Autodesk Inventor part; units mm, degrees
ref_plane "YZ Plane" through (0, 0, 0) normal (1, 0, 0) x (0, 1, 0)
ref_plane "XZ Plane" through (0, 0, 0) normal (0, 1, 0) x (-1, 0, 0)
ref_plane "XY Plane" through (0, 0, 0) normal (0, 0, 1) x (1, 0, 0)
sketch "Skizze6" plane through (0, 0, 0) normal (0, 0, 1) x (1, 0, 0)
  arc A0 (21.4454, -27.1023) -> (20.0312, -26.5165) centre (20.0312, -28.5165) ccw
  line L0 (20.0312, -26.5165) -> (-20.0312, -26.5165)
  arc A1 (-20.0312, -26.5165) -> (-21.4454, -27.1023) centre (-20.0312, -28.5165) ccw
  line L1 (-21.4454, -27.1023) -> (-51.9723, -57.6292)
  line L2 (-51.9723, -57.6292) -> (-42.4264, -67.1751)
  arc A2 (-38.3776, -89.6293) -> (-42.4264, -67.1751) centre (-56.5685, -81.3173) ccw
  arc A3 (-38.3776, -89.6293) -> (38.3776, -89.6293) centre (0, 0) ccw
  arc A4 (42.4264, -67.1751) -> (38.3776, -89.6293) centre (56.5685, -81.3173) ccw
  line L3 (42.4264, -67.1751) -> (51.9724, -57.6292)
  line L4 (51.9724, -57.6292) -> (21.4454, -27.1023)
  circle A5 centre (37.8302, -37.8302) radius 1.65
  circle A6 centre (37.8302, 37.8302) radius 1.65
  circle A7 centre (-37.8302, -37.8302) radius 1.65
  circle A8 centre (-37.8302, 37.8302) radius 1.65
  circle A9 centre (-22.7665, 22.7665) radius 1.6
  circle A10 centre (22.7665, 22.7665) radius 1.6
  circle A11 centre (22.7665, -22.7665) radius 1.6
  circle A12 centre (-22.7665, -22.7665) radius 1.6
  line L5 (19.0165, -19.0165) -> (19.0165, 19.0165)
  line L6 (19.0165, 19.0165) -> (-19.0165, 19.0165)
  line L7 (-19.0165, 19.0165) -> (-19.0165, -19.0165)
  line L8 (-19.0165, -19.0165) -> (19.0165, -19.0165)
  line L9 (26.5165, -20.8596) -> (57.6292, -51.9723)
  line L10 (57.6292, -51.9723) -> (67.1751, -42.4264)
  arc A13 (89.6293, -38.3776) -> (67.1751, -42.4264) centre (81.3173, -56.5685) ccw
  arc A14 (89.6293, -38.3776) -> (89.6293, 38.3776) centre (0, 0) ccw
  arc A15 (67.1751, 42.4264) -> (89.6293, 38.3776) centre (81.3173, 56.5685) ccw
  line L11 (67.1751, 42.4264) -> (57.6292, 51.9724)
  line L12 (57.6292, 51.9724) -> (26.5165, 20.8597)
  line L13 (26.5165, 20.8597) -> (26.5165, -20.8596)
  line L14 (-26.5165, 20.8596) -> (-57.6292, 51.9723)
  line L15 (-57.6292, 51.9723) -> (-67.1751, 42.4264)
  arc A16 (-89.6293, 38.3776) -> (-67.1751, 42.4264) centre (-81.3173, 56.5685) ccw
  arc A17 (-89.6293, 38.3776) -> (-89.6293, -38.3776) centre (0, 0) ccw
  arc A18 (-67.1751, -42.4264) -> (-89.6293, -38.3776) centre (-81.3173, -56.5685) ccw
  line L16 (-67.1751, -42.4264) -> (-57.6292, -51.9724)
  line L17 (-57.6292, -51.9724) -> (-26.5165, -20.8597)
  line L18 (-26.5165, -20.8597) -> (-26.5165, 20.8596)
  circle A19 centre (-44.3776, -92.6293) radius 1.6
  circle A20 centre (92.6293, 44.3776) radius 1.6
  circle A21 centre (-92.6293, -44.3776) radius 1.6
  circle A22 centre (44.3776, -92.6293) radius 1.6
  circle A23 centre (92.6293, -44.3776) radius 1.6
  circle A24 centre (-92.6293, 44.3776) radius 1.6
  circle A25 centre (45, 91.781) radius 1.6
  circle A26 centre (-45, 91.781) radius 1.6
  circle A27 centre (-67.8822, -48.7904) radius 1.6
  circle A28 centre (-48.7904, -67.8823) radius 1.6
  circle A29 centre (48.7904, -67.8822) radius 1.6
  circle A30 centre (67.8823, -48.7904) radius 1.6
  circle A31 centre (-67.8823, 48.7904) radius 1.6
  circle A32 centre (67.8822, 48.7904) radius 1.6
  circle A33 centre (48.7904, 67.8823) radius 1.6
  circle A34 centre (-48.7904, 67.8822) radius 1.6
  arc A35 (12, 61.781) -> (38.5642, 72.6085) centre (12, 99.781) ccw
  line L19 (12, 61.781) -> (-12, 61.781)
  arc A36 (-38.5642, 72.6085) -> (-12, 61.781) centre (-12, 99.781) ccw
  arc A37 (-42.4264, 67.1751) -> (-38.5642, 72.6085) centre (-56.5685, 81.3173) ccw
  line L20 (-42.4264, 67.1751) -> (-51.9724, 57.6292)
  line L21 (-51.9724, 57.6292) -> (-20.8597, 26.5165)
  line L22 (-20.8597, 26.5165) -> (20.8596, 26.5165)
  line L23 (20.8596, 26.5165) -> (51.9723, 57.6292)
  line L24 (51.9723, 57.6292) -> (42.4264, 67.1751)
  arc A38 (38.5642, 72.6085) -> (42.4264, 67.1751) centre (56.5685, 81.3173) ccw
  line L25 (-12, 71.781) -> (12, 71.781)
  arc A39 (12, 71.781) -> (39.8653, 97.0378) centre (12, 99.781) ccw
  arc A40 (42.6492, 98.6778) -> (39.8653, 97.0378) centre (41.8557, 96.8419) ccw
  arc A41 (50.5184, 94.8902) -> (42.6492, 98.6778) centre (0, 0) ccw
  arc A42 (51.2299, 90.1207) -> (50.5184, 94.8902) centre (49.1086, 92.2421) ccw
  line L26 (51.2299, 90.1207) -> (49.4975, 88.3883)
  arc A43 (49.4975, 88.3883) -> (49.4975, 74.2462) centre (56.5685, 81.3173) ccw
  line L27 (49.4975, 74.2462) -> (74.2462, 49.4975)
  arc A44 (74.2462, 49.4975) -> (88.3884, 49.4975) centre (81.3173, 56.5685) ccw
  line L28 (88.3884, 49.4975) -> (90.1208, 51.2299)
  arc A45 (94.8902, 50.5184) -> (90.1208, 51.2299) centre (92.2421, 49.1086) ccw
  arc A46 (94.8902, -50.5184) -> (94.8902, 50.5184) centre (0, 0) ccw
  arc A47 (90.1208, -51.2299) -> (94.8902, -50.5184) centre (92.2421, -49.1086) ccw
  line L29 (90.1208, -51.2299) -> (88.3883, -49.4975)
  arc A48 (88.3883, -49.4975) -> (74.2462, -49.4975) centre (81.3173, -56.5685) ccw
  line L30 (74.2462, -49.4975) -> (49.4975, -74.2462)
  arc A49 (49.4975, -74.2462) -> (49.4975, -88.3883) centre (56.5685, -81.3173) ccw
  line L31 (49.4975, -88.3883) -> (51.2299, -90.1207)
  arc A50 (50.5184, -94.8902) -> (51.2299, -90.1207) centre (49.1086, -92.2421) ccw
  arc A51 (-50.5184, -94.8902) -> (50.5184, -94.8902) centre (0, 0) ccw
  arc A52 (-51.2299, -90.1208) -> (-50.5184, -94.8902) centre (-49.1086, -92.2421) ccw
  line L32 (-51.2299, -90.1208) -> (-49.4975, -88.3883)
  arc A53 (-49.4975, -88.3883) -> (-49.4975, -74.2462) centre (-56.5685, -81.3173) ccw
  line L33 (-49.4975, -74.2462) -> (-74.2462, -49.4975)
  arc A54 (-74.2462, -49.4975) -> (-88.3883, -49.4975) centre (-81.3173, -56.5685) ccw
  line L34 (-88.3883, -49.4975) -> (-90.1207, -51.2299)
  arc A55 (-94.8902, -50.5184) -> (-90.1207, -51.2299) centre (-92.2421, -49.1086) ccw
  arc A56 (-94.8902, 50.5184) -> (-94.8902, -50.5184) centre (0, 0) ccw
  arc A57 (-90.1208, 51.2299) -> (-94.8902, 50.5184) centre (-92.2421, 49.1086) ccw
  line L35 (-90.1208, 51.2299) -> (-88.3883, 49.4975)
  arc A58 (-88.3883, 49.4975) -> (-74.2462, 49.4975) centre (-81.3173, 56.5685) ccw
  line L36 (-74.2462, 49.4975) -> (-49.4975, 74.2462)
  arc A59 (-49.4975, 74.2462) -> (-49.4975, 88.3883) centre (-56.5685, 81.3173) ccw
  line L37 (-49.4975, 88.3883) -> (-51.2299, 90.1207)
  arc A60 (-50.5184, 94.8902) -> (-51.2299, 90.1207) centre (-49.1086, 92.2421) ccw
  arc A61 (-42.6492, 98.6778) -> (-50.5184, 94.8902) centre (0, 0) ccw
  arc A62 (-39.8653, 97.0378) -> (-42.6492, 98.6778) centre (-41.8557, 96.8419) ccw
  arc A63 (-39.8653, 97.0378) -> (-12, 71.781) centre (-12, 99.781) ccw
  arc A64 (-47.6003, 86.4911) -> (-12, 61.781) centre (-12, 99.781) ccw
  line L38 (-49.4975, 88.3883) -> (-47.6003, 86.4911)
  line L39 (0, 71.781) -> (0, 61.781) construction
  arc A65 (12, 61.781) -> (47.6003, 86.4911) centre (12, 99.781) ccw
  line L40 (49.4975, 88.3883) -> (47.6003, 86.4911)
  point P0 (0, 0)
  point P1 (0, 0)
  point P2 (38.5642, 72.6085)
extrude "Extrusion4" add sketch "Skizze6" against normal blind 30 contours L19 A36 A64 L38 L37 A60 A61 A62 A63 L25 A39 A40 A41 A42 L26 L40 A65 A35
fillet "Rundung2" radius 20 2 edges at (47.6003, 86.4911, -15) (-47.6003, 86.4911, -15)
sketch "Skizze7" plane through (0, 0, 0) normal (0, 0, 1) x (1, 0, 0)
  line L0 (0, 0) -> (-29.0841, 0) construction
  line L1 (0, 0) -> (-84.8528, 84.8528)
  line L2 (-111.3693, 68.9429) -> (-68.9429, 111.3693)
  line L3 (-68.9429, 111.3693) -> (-58.3363, 100.7627)
  line L4 (-58.3363, 100.7627) -> (-100.7627, 58.3363)
  line L5 (-100.7627, 58.3363) -> (-111.3693, 68.9429)
  line L6 (-111.3693, 68.9429) -> (-58.3363, 100.7627) construction
  line L7 (-68.9429, 111.3693) -> (-100.7627, 58.3363) construction
  dimension "d19" = 45
  dimension "d20" = 120
  dimension "d21" = 60
  dimension "d22" = 15
extrude "Extrusion5" add sketch "Skizze7" against normal blind 30
sketch "Skizze8" plane through (-68.9429, 111.3693, -30) normal (-0.7071, 0.7071, 0) x (-0.7071, -0.7071, 0)
  line L0 (60, 0) -> (0, 0)
  line L1 (30, 0) -> (30, 17.5)
  circle A0 centre (30, 17.5) radius 30
  line L2 (0, 30) -> (60, 30)
  line L3 (0, 30) -> (60, 30)
  line L4 (60, 30) -> (60, 0)
  line L5 (60, 0) -> (0, 0)
  line L6 (0, 0) -> (0, 30)
  point P0 (30, 30)
  dimension "d25" = 17.5
  dimension "d26" = 60
extrude "Extrusion6" cut sketch "Skizze8" against normal up to surface (15 mm away) contours L0 A0 L4 | L0 A0 L2 | A0 L2 L4 | L0 L6 A0 | L6 L2 A0
extrude "Extrusion7" cut sketch "Skizze8" against normal blind 100 contours A0 L0 | L0 A0 L2 | L2 A0
mirror "Spiegeln1" about plane through (0, 0, 0) normal (1, 0, 0) of "Extrusion7"
sketch "Skizze9" plane through (0, 0, 0) normal (0, 0, 1) x (1, 0, 0)
  circle A0 centre (45, 91.781) radius 1.6
  circle A1 centre (45, 91.781) radius 2.1
  circle A2 centre (-45, 91.781) radius 1.6
  circle A3 centre (-45, 91.781) radius 2.1
  point P0 (0, 0)
  dimension "d31" = 4.2
  dimension "d32" = 4.2
extrude "Extrusion8" cut sketch "Skizze9" against normal up to surface (30 mm away) contours A0 | A1 | A2 | A3
properties part number "Ballkuhle"
Verification items for the finished model (mm, model axes). A direction names the side the tool comes from. Coordinates: 2 decimals unless noted, no trailing zeros. Order: outer loops, then holes, each group sorted by start corner. A loop starts at its lowest first (then second) coordinate and runs counter-clockwise, first axis right, second up. Notation, with made-up numbers: (-21, -14) -> (33, -14) arc R14 cw to (33, 10) -> close; hole circle Ø11 at (48, -17). An arc over 180 degrees is marked (long way). Put each result on its own line as item: value. Start each with the question number.
1) Material ranges on L1, parallel to X at y = 91, z = -27; L2, parallel to Z at x = 45, y = 85.5; L3, parallel to X at y = 94, z = -22, recorded low to high.
2) Tool access check on faces 4 (the flat face through (0, 61.781, -15)), 5 (the cylindrical face through (30.589, 78.842, -14.79)). Record the directions out of +Z, -Z, +X, -X, +Y, -Y that give a thin tool (end or side, any length) a straight path to the whole face; none if there is none.
3) Cross-section at B-B (z = -20.5). Enter the section's corners in (x, y).
4) Go/stop test with flat-tipped pins: pin 1 (4 mm diameter, centred on x = -16.5, z = -3.5, fed in from +Y); pin 2 (2 mm diameter, centred on y = 84, z = -26.5, fed in from -X); pin 3 (2.5 mm diameter, centred on x = 45, y = 91.781, fed in from +Z); pin 4 (4 mm diameter, centred on y = 73.5, z = -17, fed in from +X). Record where each tip stops, or that it passes through.
5) Release check for a two-part mould opening along Y. For faces 1 (the cylindrical face through (-44.03, 89.92, -14.79)), 2 (the cylindrical face through (-19.1, 62.45, -14.79)), 3 (the flat face through (0, 71.781, -15)) record: pulls with the +Y half, pulls with the -Y half, needs draft (parallel to the pull), parting line crosses it, or undercut.
6) Cross-section at A-A (z = -10.5). Enter the section's corners in (x, y).
7) Cross-section at C-C (x = 1.5). Enter the section's corners in (y, z).
Geometry check:
1. L1: x = -51.84 to -46.95, -43.05 to -38.59, 38.59 to 43.05, 46.95 to 51.84
1. L2: z = -30 to -21.44, -3.56 to 0
1. L3: x = -51.54 to -39.4, 39.4 to 51.54
2. face 4: +Z, -Z, +X, -X, -Y
2. face 5: +Z, -Z, +Y
3. outline: (-52.03, 92.92) -> (-22.32, 63.21) arc R38 ccw to (-12, 61.78) -> (12, 61.78) arc R38 ccw to (22.32, 63.21) -> (52.03, 92.92) arc R3 ccw to (50.52, 94.89) arc R107.51 ccw to (42.65, 98.68) arc R2 ccw to (39.87, 97.04) arc R28 cw to (12, 71.78) -> (-12, 71.78) arc R28 cw to (-39.87, 97.04) arc R2 ccw to (-42.65, 98.68) arc R107.49 ccw to (-50.52, 94.89) arc R3 ccw to start; hole circle Ø4.2 at (-45, 91.78); hole circle Ø4.2 at (45, 91.78)
4. pin 1: stops at y = 72.55
4. pin 2: stops at x = -47.11
4. pin 3: passes through
4. pin 4: stops at x = 33.6
5. face 1: undercut
5. face 2: pulls with the -Y half
5. face 3: pulls with the +Y half
6. outline: (-51.59, 93.92) -> (-20.39, 62.72) arc R38 ccw to (-12, 61.78) -> (12, 61.78) arc R38 ccw to (20.39, 62.72) -> (51.59, 93.92) arc R3 ccw to (50.52, 94.89) arc R107.51 ccw to (42.65, 98.68) arc R2 ccw to (39.87, 97.04) arc R28 cw to (12, 71.78) -> (-12, 71.78) arc R28 cw to (-39.87, 97.04) arc R2 ccw to (-42.65, 98.68) arc R107.49 ccw to (-50.52, 94.89) arc R3 ccw to start; hole circle Ø4.2 at (-45, 91.78); hole circle Ø4.2 at (45, 91.78)
7. outline: (61.78, -30) -> (71.78, -30) -> (71.78, 0) -> (61.78, 0) -> close
